Source: CAD feature listing. Evaluate the final solid. Frame: model axes, mm. Face numbers are marked on the shaded views. A direction names the side the tool comes from. Coordinates: 2 decimals unless noted, no trailing zeros. Write each loop counter-clockwise with the first axis right and the second up, starting at its lowest first coordinate (ties: lowest second). Pieces come first, ordered by that corner, then holes. Notation, with made-up numbers: (86.25, 77.25) -> (127.25, 77.25) arc R27 cw to (127.25, 115.25) -> close; hole circle Ø4 at (-6.5, 46). An arc over 180 degrees is marked (long way). Write item = value, one per line.
from build123d import *

# Parameters (mm, degrees)
F0_R     = 11
F0_R_2   = 3.7
F1_DEPTH = 4
F2_DEPTH = 7
F3_SIZE  = 3.99999
F4_SIZE  = 1


# Not quite as in the source:
# - a fillet or chamfer is up to 0.001 mm smaller than in the source, because OpenCascade refuses the exact size


with BuildPart() as f1:
    # F0 (on Top) → F1 (new body)
    with BuildSketch(Plane.XY):
        Circle(F0_R)
        Circle(F0_R_2, mode=Mode.SUBTRACT)
        Circle(F0_R_2)
    extrude(amount=F1_DEPTH)

    # F0 (on Top) → F2 (join)
    with BuildSketch(Plane.XY):
        Circle(F0_R_2)
    extrude(amount=F2_DEPTH)

    # F3 (size 4 in the source; OpenCascade refuses exactly that, so slightly less here)
    f3_edges = [f1.edges().sort_by_distance(p)[0] for p in [
        (-11, 0, 0),
    ]]
    chamfer(f3_edges, length=F3_SIZE)

    # F4
    f4_edges = [f1.edges().sort_by_distance(p)[0] for p in [
        (-3.7, 0, 4),
    ]]
    chamfer(f4_edges, length=F4_SIZE)


solid = f1.part
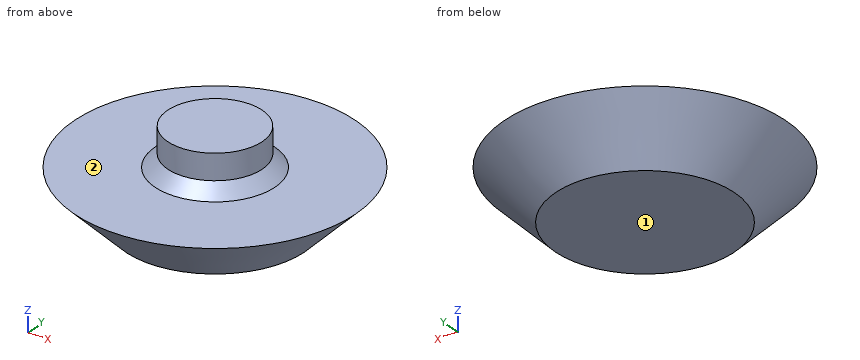
1) First-contact query: pin 1 Ø4 at (y, z) = (5.5, 1.5) entering from +X; pin 2 Ø3 at (x, y) = (-5.5, 5) entering from -Z; pin 3 Ø1 at (y, z) = (2, 5.5) entering from -X; pin 4 Ø5 at (x, y) = (-7, 6) entering from +Z. Flat tips, straight axial feed; report the tip coordinate or a pass-through.
Answer block:
pin_1 = 9.2
pin_2 = 0
pin_3 = -3.38
pin_4 = 4
2) Cut plane C-C, the plane z = 4.5. Output: boundary loops of the cut face in (x, y).
Answer block:
outline = circle Ø8.4 at (0, 0)
3) Material intervals for probe 1 along Z at (x, y) = (5.75, -1); probe 2 along Y at (x, z) = (0, 6.25); probe 3 along Z at (x, y) = (-9.25, 1.5), sorted ascending. Write a range as [from, to].
Answer block:
probe_1 = [0, 4]
probe_2 = [-3.7, 3.7]
probe_3 = [2.37, 4]
4) Cut plane D-D, the plane z = 1.5. Output: boundary loops of the cut face in (x, y), and give its area (3 significant figures).
Answer block:
outline = circle Ø17 at (0, 0)
area = 227 mm2
5) Reachability of the marked faces 1 and 2 from +Z, -Z, +X, -X, +Y, -Y: full face, straight path, thin tool, end or side. Return the list, or none.
Answer block:
face_1 = -Z, +X, -X, +Y, -Y
face_2 = +Z
